```python
from build123d import *

# Parameters (mm, degrees)
SKETCH_W      = 4
SKETCH_H      = 12
SKETCH_R      = 1.6
PAD_DEPTH     = 12
SKETCH001_R   = 1.6
SKETCH001_R_2 = 1.5
PAD001_DEPTH  = 5
SKETCH002_W   = 14
SKETCH002_H   = 12
SKETCH002_R   = 1
SKETCH002_R_2 = 2.5
POCKET_DEPTH  = 3.001
SKETCH003_W   = 2
SKETCH003_H   = 1.5
PAD002_DEPTH  = 12
CHAMFER_SIZE  = 1.99
FILLET002_R   = 2
FILLET_R      = 3


with BuildPart() as part:
    # Sketch → Pad (new body)
    with BuildSketch(Plane.XY):
        with Locations((2, 6)):
            Rectangle(SKETCH_W, SKETCH_H)
        with Locations((2, 6)):
            Circle(SKETCH_R, mode=Mode.SUBTRACT)
    extrude(amount=PAD_DEPTH)

    # Sketch001 → Pad001 (join)
    with BuildSketch(Plane.XY):
        Polygon((0, -4), (4, -4), (4, 0), (19, 0), (19, 12), (4, 12), (4, 16), (0, 16), align=None)
        with Locations((2, 6)):
            Circle(SKETCH001_R, mode=Mode.SUBTRACT)
        with Locations((9, 6)):
            Circle(SKETCH001_R_2, mode=Mode.SUBTRACT)
    extrude(amount=-PAD001_DEPTH)

    # Sketch002 (on DatumPlane) → Pocket (cut, through all)
    with BuildSketch(Plane.XY.offset(-2)):
        with Locations((12, 6)):
            Rectangle(SKETCH002_W, SKETCH002_H)
        with Locations((14, 9.1)):
            Circle(SKETCH002_R, mode=Mode.SUBTRACT)
        with Locations((14, 2.9)):
            Circle(SKETCH002_R, mode=Mode.SUBTRACT)
        with Locations((9, 6)):
            Circle(SKETCH002_R_2, mode=Mode.SUBTRACT)
    extrude(amount=-POCKET_DEPTH, mode=Mode.SUBTRACT)

    # Sketch003 → Pad002 (join)
    with BuildSketch(Plane.XY):
        with Locations((5, 9.25)):
            Rectangle(SKETCH003_W, SKETCH003_H)
        with Locations((5, 2.75)):
            Rectangle(SKETCH003_W, SKETCH003_H)
    extrude(amount=PAD002_DEPTH)

    # Chamfer
    chamfer_edges = [part.edges().sort_by_distance(p)[0] for p in [
        (6, 2.75, 12),
        (6, 9.25, 12),
    ]]
    chamfer(chamfer_edges, length=CHAMFER_SIZE)

    # Fillet002
    fillet002_edges = [part.edges().sort_by_distance(p)[0] for p in [
        (4, 6, 0),
    ]]
    fillet(fillet002_edges, radius=FILLET002_R)

    # Fillet
    fillet_edges = [part.edges().sort_by_distance(p)[0] for p in [
        (19, 0, -1),
        (19, 12, -1),
    ]]
    fillet(fillet_edges, radius=FILLET_R)


solid = part.part
```
Could you check a few things on this model? Use its own coordinates, in mm. A direction names the side the tool comes from. Coordinates: 2 decimals unless noted, no trailing zeros. Loops run counter-clockwise (first coordinate to the right, second up) from the corner with the lowest first, then second, coordinate; pieces in that order, holes last.
1) Will these pins go through, and if not, where does the flat tip stop? pin 1 Ø2.5 at (x, z) = (11, -3) entering from -Y; pin 2 Ø1.2 at (y, z) = (15, -3) entering from +X; pin 3 Ø1.2 at (y, z) = (3, 4) entering from +X.
Reported:
pin 1: stops at y = 0
pin 2: stops at x = 4
pin 3: stops at x = 6
2) Imagine slicing it at D-D (z = 11.25). List the corners of the cut face in (x, y) for me.
Reported:
outline: (0, 0) - (4, 0) - (4, 2) - (4.76, 2) - (4.76, 3.5) - (4, 3.5) - (4, 8.5) - (4.76, 8.5) - (4.76, 10) - (4, 10) - (4, 12) - (0, 12) - close; hole circle Ø3.2 at (2, 6)
3) Imagine slicing it at C-C (x = 2). List the corners of the cut face in (y, z) for me, and give its area (3 significant figures).
Reported:
outline: (-4, -5) - (4.4, -5) - (4.4, 12) - (0, 12) - (0, 0) - (-4, 0) - close; (7.6, -5) - (16, -5) - (16, 0) - (12, 0) - (12, 12) - (7.6, 12) - close
area: 190 mm2
4) Please list where these lines run through material, in increasing order: line 1 along Y through (x, z) = (9, -3.2); line 2 along Y through (x, z) = (5.25, 2.5); line 3 along Z through (x, y) = (1.5, 14.25).
Reported:
line 1: y = 3.5 to 4.5, 7.5 to 8.5
line 2: y = 2 to 3.5, 8.5 to 10
line 3: z = -5 to 0
5) Which directions (+Z, -Z, +X, -X, +Y, -Y) give clear straight access to the entire face, cutting with the end or side of a thin tool? Please do faces 1 (the face through (4, 1, 6)), 2 (the face through (4, -2, -2)), 3 (the face through (4, 14, -2)), 4 (the face through (6, 9, 5)), 5 (the face through (5, 3.5, 6)).
Reported:
face 1: +Z, +X, -Y
face 2: +Z, -Z, +X, -Y
face 3: +Z, -Z, +X, +Y
face 4: +Z, +X, +Y, -Y
face 5: +Z, +X
6) Imagine slicing it at A-A (y = 6). List the corners of the cut face in (x, z) for me.
Reported:
outline: (0, -5) - (0.4, -5) - (0.4, 12) - (0, 12) - close; (3.6, -5) - (5, -5) - (5, -2) - (6.5, -2) - (6.5, -5) - (7.5, -5) - (7.5, 0) - (6, 0) arc R2 cw to (4, 2) - (4, 12) - (3.6, 12) - close; (10.5, -5) - (11.5, -5) - (11.5, -2) - (19, -2) - (19, 0) - (10.5, 0) - close
7) Imagine slicing it at B-B (z = -1). List the corners of the cut face in (x, y) for me, and give its area (3 significant figures).
Reported:
outline: (0, -4) - (4, -4) - (4, 0) - (16, 0) arc R3 ccw to (19, 3) - (19, 9) arc R3 ccw to (16, 12) - (4, 12) - (4, 16) - (0, 16) - close; hole circle Ø3.2 at (2, 6); hole circle Ø3 at (9, 6)
area: 241 mm2
8) Thinking about a two-plate mould opening in Y: for faces 6 (the face through (18.1, 11.14, -1.01)), 7 (the face through (7.8, 5.1, -2.5)), 8 (the face through (5, 6, -3)), 9 (the face through (10, 0, -1)), which applies, released by +Y, released by -Y, zero draft, split by the parting line, or undercut?
Reported:
face 6: released by +Y
face 7: undercut
face 8: zero draft
face 9: released by -Y
